```python
from build123d import *

# Parameters (mm, degrees)
SKETCH_1_W          = 6
SKETCH_1_H          = 6
EXTRUDE_1_DEPTH     = 10
SKETCH_2_W          = 2.4
SKETCH_2_H          = 8
CUT_EXTRUDE_1_DEPTH = 10
SKETCH_3_RX         = 6
SKETCH_3_RY         = 4.5
EXTRUDE_2_DEPTH     = 2.5
SKETCH_4_RX         = 3.5
SKETCH_4_RY         = 3
CUT_EXTRUDE_3_DEPTH = 2.5
CUT_EXTRUDE_4_DEPTH = 2


with BuildPart() as part:
    # 草图1 → 凸台-拉伸1 (new body)
    with BuildSketch(Plane(origin=(0, 0, 0), x_dir=(1, 0, 0), z_dir=(0, 1, 0))):
        with Locations((-2.112149533, 1.495327103)):
            Rectangle(SKETCH_1_W, SKETCH_1_H)
    extrude(amount=EXTRUDE_1_DEPTH)

    # 草图2 → 切除-拉伸1 (cut)
    with BuildSketch(Plane.XY.offset(1.504672897)):
        with Locations((-2.112149533, 4)):
            Rectangle(SKETCH_2_W, SKETCH_2_H)
    extrude(amount=-CUT_EXTRUDE_1_DEPTH, mode=Mode.SUBTRACT)

    # 草图3 → 凸台-拉伸2 (add)
    with BuildSketch(Plane(origin=(0.887850467, 0, 0), x_dir=(0, 0, -1), z_dir=(1, 0, 0))):
        with Locations(Location((1.495327103, 5), (0, 0, 0))):
            Ellipse(SKETCH_3_RX, SKETCH_3_RY)
    extrude(amount=EXTRUDE_2_DEPTH)

    # 草图4 → 切除-拉伸3 (cut)
    with BuildSketch(Plane(origin=(3.387850467, 0, 0), x_dir=(0, 0, -1), z_dir=(1, 0, 0))):
        with Locations(Location((1.495327103, 5), (0, 0, 180))):
            Ellipse(SKETCH_4_RX, SKETCH_4_RY)
    extrude(amount=-CUT_EXTRUDE_3_DEPTH, mode=Mode.SUBTRACT)

    # 草图5 → 切除-拉伸4 (cut)
    with BuildSketch(Plane(origin=(0.887850467, 0, 0), x_dir=(0, 0, -1), z_dir=(1, 0, 0))):
        with BuildLine():
            Line((-0.467124992, 5.741987188), (3.424164273, 5.741987188))
            ThreePointArc((3.424164273, 5.741987188), (4.166151461, 5), (3.424164273, 4.258012812))
            Line((3.424164273, 4.258012812), (-0.467124992, 4.258012812))
            ThreePointArc((-0.467124992, 4.258012812), (-1.20911218, 5), (-0.467124992, 5.741987188))
        make_face()
    extrude(amount=-CUT_EXTRUDE_4_DEPTH, mode=Mode.SUBTRACT)


solid = part.part
```
Model file for the job. Use its own axes, mm. A direction names the side the tool comes from. Give positions to 0.01 mm unless a question says otherwise; leave off trailing zeros. Order: outer loops, then holes, each group sorted by start corner. A loop starts at its lowest first (then second) coordinate and runs counter-clockwise, first axis right, second up.
1) Saw through at A-A, the plane x = -2.25. Write the cut outline in (y, z).
2) Wall check: probe 1 along X at (y, z) = (7.25, -0.25); probe 2 along X at (y, z) = (7.75, -3.5); probe 3 along Z at (x, y) = (0.5, 3.75). Give the ranges that are in metal, low to high.
3) Mould opens along X. For faces 1 (the flat face through (-0.912, 4, -1)), 2 (the flat face through (3.388, 2, -3)), 3 (the flat face through (0, 5.742, -1)) say: +X half, -X half, draft (parallel to the pull), parting line (faces both ways), or undercut.
4) 3-axis set-ups, long thin cutter, end or side, ignore diameter. For faces 4 (the flat face through (-3.5, 4.9, 1.505)), 5 (the flat face through (0.888, 0.3, -1.5)), 6 (the flat face through (0.888, 9.7, -1.5)), 7 (the cylindrical face through (0, 4.98, 1.21)): which of +Z, -Z, +X, -X, +Y, -Y reach the whole face in a straight line?
5) Saw through at B-B, the plane y = 5. Count the separate pieces of the cut face and the enclosed holes in it, then the cut area to 3 significant figures.
6) Pin check, flat tips, straight feed: pin 1 (1.2 mm diameter, centred on x = -2.5, z = -1.5, fed in from -Y); pin 2 (2.5 mm diameter, centred on y = 3, z = 3, fed in from -X); pin 3 (4 mm diameter, centred on x = -1.5, y = 5, fed in from -Z). Stop position of each tip, or through.
Computed:
1. outline: (8, -4.5) - (10, -4.5) - (10, 1.5) - (8, 1.5) - close
2. probe 1: x = -5.11 to -3.31, -0.91 to 0.89
2. probe 2: x = -5.11 to -3.31, -0.91 to 3.39
2. probe 3: z = -4.5 to 1.5
3. face 1: undercut
3. face 2: +X half
3. face 3: draft
4. face 4: +Z, -X, +Y, -Y
4. face 5: +X, -Y
4. face 6: +X, +Y
4. face 7: +X
5. separate pieces: 5
5. enclosed holes: 0
5. area: 24.4 mm2
6. pin 1: stops at y = 8
6. pin 2: stops at x = 0.89
6. pin 3: stops at z = -4.5
